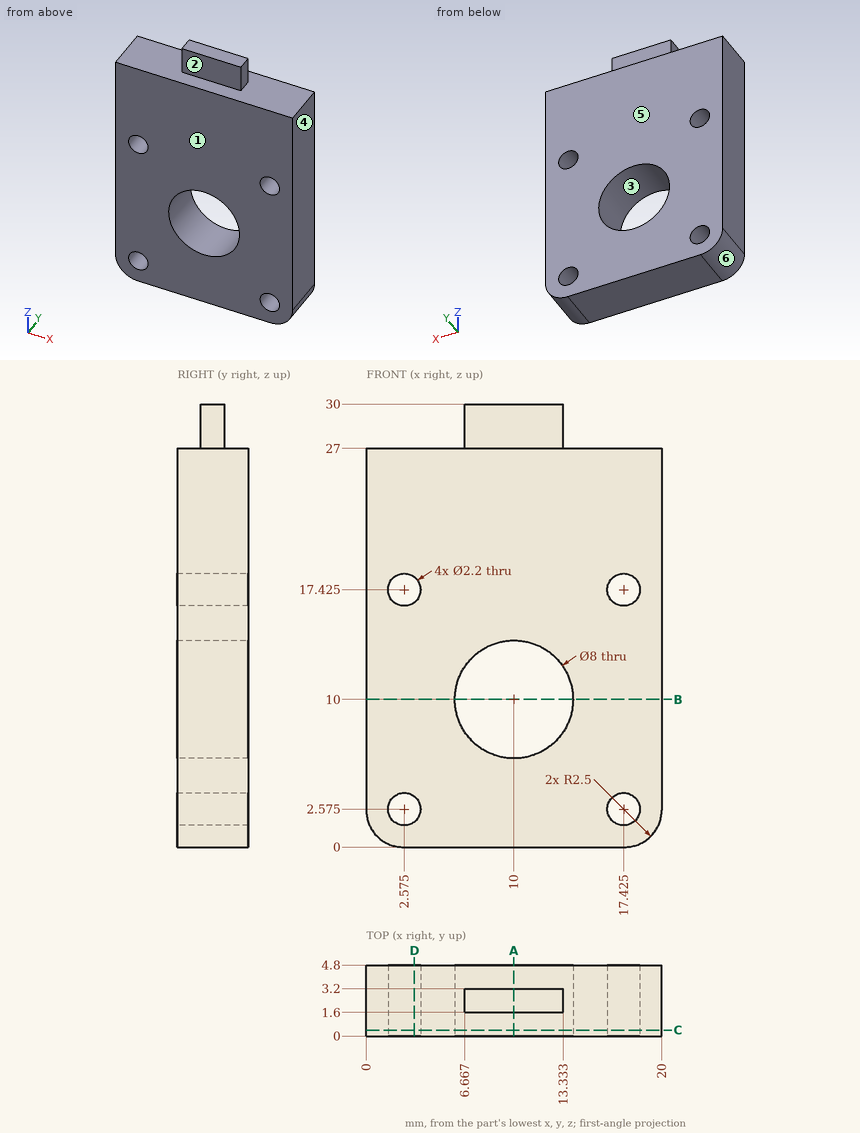
Study the drawing (mm; zero at the part's minimum x, y, z) and answer. A direction names the side the tool comes from. Round coordinates to 2 decimals unless told otherwise and drop trailing zeros. Write each loop counter-clockwise with the first axis right and the second up, starting at its lowest first coordinate (ties: lowest second). Pieces come first, ordered by that corner, then holes. Notation, with made-up numbers: (72, 70.25) -> (99, 70.25) arc R11 cw to (99, 81.25) -> close; hole circle Ø11 at (32.5, -39). An arc over 180 degrees is marked (long way). Answer as CSV lines item,"result". Start each with the question number.
(1) Each of these flat-tipped pins is pushed along its axis until it touches: pin 1 (0.8 mm diameter, centred on y = 2.5, z = 29, fed in from -X); pin 2 (0.5 mm diameter, centred on y = 2.5, z = 28, fed in from +X); pin 3 (1.8 mm diameter, centred on x = 17.42, z = 2.58, fed in from -Y); pin 4 (1.5 mm diameter, centred on x = 8.5, z = 28, fed in from -Y). Where does it stop, or does it pass through?
(2) The mould has two halves that part along X. Classify the marked faces 3, 4, 5 and 6: +X half, -X half, draft (parallel to the pull), parting line (faces both ways), or undercut.
(3) The part is cut by section C-C, the plane y = 0.4. Give the vertices of the cut face in (x, z) (1 decimal), then the cut area to 3 significant figures.
(4) The part is cut by section B-B, the plane z = 10. Give the vertices of the cut face in (x, y), then the cut area to 3 significant figures.
(5) Find the intervals of material crossed by probe 1 along X at (y, z) = (4, 17); probe 2 along X at (y, z) = (3.65, 2.25) (1 decimal); probe 3 along Z at (x, y) = (3.5, 1.8), in increasing order.
(6) A tool of negligible diameter and unlimited length cuts with its end or side. For the marked faces 1 and 2, from which of +Z, -Z, +X, -X, +Y, -Y can it reach the whole face along a straight path? Write none if from no direction.
(7) The part is cut by section A-A, the plane x = 10. Give the vertices of the cut face in (y, z).
(8) The part is cut by section D-D, the plane x = 3.25. Give the vertices of the cut face in (y, z).
Output values:
1,pin 1,"stops at x = 6.67"
1,pin 2,"stops at x = 13.33"
1,pin 3,"passes through"
1,pin 4,"stops at y = 1.6"
2,face 3,"undercut"
2,face 4,"+X half"
2,face 5,"draft"
2,face 6,"-X half"
3,outline,"(0, 2.5) arc R2.5 ccw to (2.5, 0) -> (17.5, 0) arc R2.5 ccw to (20, 2.5) -> (20, 27) -> (0, 27) -> close; hole circle Ø2.2 at (2.6, 2.6); hole circle Ø2.2 at (2.6, 17.4); hole circle Ø8 at (10, 10); hole circle Ø2.2 at (17.4, 2.6); hole circle Ø2.2 at (17.4, 17.4)"
3,area,"472 mm²"
4,outline,"(0, 0) -> (6, 0) -> (6, 4.8) -> (0, 4.8) -> close; (14, 0) -> (20, 0) -> (20, 4.8) -> (14, 4.8) -> close"
4,area,"57.6 mm²"
5,probe 1,"x = 0 to 1.56, 3.59 to 16.41, 18.44 to 20"
5,probe 2,"x = 0 to 1.5, 3.6 to 16.4, 18.5 to 20"
5,probe 3,"z = 0 to 1.98, 3.17 to 16.83, 18.02 to 27"
6,face 1,"+Z, -Z, +X, -X, -Y"
6,face 2,"+Z, +X, -X, -Y"
7,outline,"(0, 0) -> (4.8, 0) -> (4.8, 6) -> (0, 6) -> close; (0, 14) -> (4.8, 14) -> (4.8, 27) -> (3.2, 27) -> (3.2, 30) -> (1.6, 30) -> (1.6, 27) -> (0, 27) -> close"
8,outline,"(0, 0) -> (4.8, 0) -> (4.8, 1.71) -> (0, 1.71) -> close; (0, 3.44) -> (4.8, 3.44) -> (4.8, 16.56) -> (0, 16.56) -> close; (0, 18.29) -> (4.8, 18.29) -> (4.8, 27) -> (0, 27) -> close"
